Input: part model. Units: mm. Frame: model coordinates. Face numbers are marked on the shaded views. A direction names the side the tool comes from. Give positions to 0.01 mm unless a question says otherwise; leave off trailing zeros. Loops run counter-clockwise (first coordinate to the right, second up) from the corner with the lowest first, then second, coordinate; pieces in that order, holes last. Notation, with made-up numbers: M 87,37.5 L 109,37.5 A30 ccw 109,71.5 Z; hole C -6.75,47 d2. An arc over 180 degrees is marked long. Answer as a JSON object with one key per item and string values. Group by question number.
1) Section query D-D on x = -30. Return loops of the section in (y, z).
2) Draft query along Y for the marked faces 1, 2, 3 and 4. Return one class per face: +Y half, -Y half, draft (parallel to the pull), parting line (faces both ways), or undercut.
3) Section query C-C on x = 23. Return loops of the section in (y, z), plus the area to 3 significant figures.
4) Section query B-B on y = -8. Return loops of the section in (x, z).
5) First-contact query: P1, Ø18, axis at x = 18, y = -7, coming from the +Z side; P2, Ø16, axis at x = 23, y = 0, coming from the +Z side. Flat tips, straight axial feed; report the tip coordinate or a pass-through.
6) Ray query, L1, parallel to Y at x = 23, z = 38.75; L2, parallel to Z at x = -24, y = 11.5; L3, parallel to Z at x = 29, y = -0.5. Return the intervals inside material, ascending.
7) Access query for the marked faces 5 and 6. Directions: +Z, -Z, +X, -X, +Y, -Y. A direction counts if a zero-diameter tool reaches every point of the face in a straight line with its end or side. Return the directions, or none.
8) Section query A-A on z = 38. Return loops of the section in (x, y).
from build123d import *

# Parameters (mm, degrees)
F0_W     = 80
F0_H     = 60
F1_DEPTH = 50
F2_R     = 10
F3_DEPTH = 18.5
F4_R     = 10
F5_DEPTH = 20


with BuildPart() as f1:
    # F0 (on Top) → F1 (new body)
    with BuildSketch(Plane.XY):
        Rectangle(F0_W, F0_H)
    extrude(amount=F1_DEPTH)

    # F2 (on face) → F3 (join)
    with BuildSketch(Plane.XY.offset(50)):
        with Locations((-30, 0)):
            Circle(F2_R)
    extrude(amount=F3_DEPTH)

    # F4 (on face) → F5 (cut)
    with BuildSketch(Plane.XY.offset(50)):
        with Locations((23, 0)):
            Circle(F4_R)
    extrude(amount=-F5_DEPTH, mode=Mode.SUBTRACT)


solid = f1.part
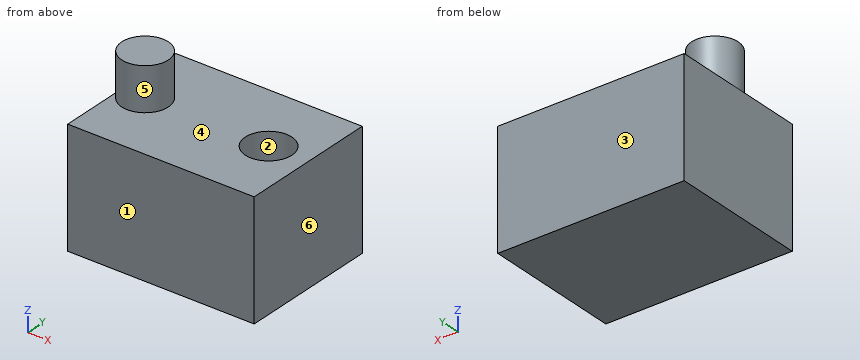
Output:
{
 "1": {"outline": "M -30,0 L 30,0 L 30,50 L 10,50 L 10,68.5 L -10,68.5 L -10,50 L -30,50 Z"},
 "2": {"face 1": "-Y half", "face 2": "undercut", "face 3": "+Y half", "face 4": "draft"},
 "3": {"outline": "M -30,0 L 30,0 L 30,50 L 10,50 L 10,30 L -10,30 L -10,50 L -30,50 Z", "area": "2,600 mm^2"},
 "4": {"outline": "M -40,0 L 40,0 L 40,50 L 29,50 L 29,30 L 17,30 L 17,50 L -24,50 L -24,68.5 L -36,68.5 L -36,50 L -40,50 Z"},
 "5": {"P1": "stops at z = 50", "P2": "stops at z = 30"},
 "6": {"L1": "y = -30 to -10, 10 to 30", "L2": "z = 0 to 50", "L3": "z = 0 to 30"},
 "7": {"face 5": "+Z", "face 6": "+Z, -Z, +X, +Y, -Y"},
 "8": {"outline": "M -40,-30 L 40,-30 L 40,30 L -40,30 Z; hole C 23,0 d20"}
}
